Autodesk Inventor part; units mm, degrees
ref_plane "YZ Plane" through (0, 0, 0) normal (1, 0, 0) x (0, 1, 0)
ref_plane "XZ Plane" through (0, 0, 0) normal (0, 1, 0) x (-1, 0, 0)
ref_plane "XY Plane" through (0, 0, 0) normal (0, 0, 1) x (1, 0, 0)
sketch "Sketch1" plane through (0, 0, 0) normal (0, 1, 0) x (-1, 0, 0)
  line L0 (100, 100.3504) -> (-94, 100.3504)
  line L1 (94, -100) -> (94, -50)
  line L2 (94, -50) -> (100, -50)
  line L3 (100, 0) -> (94, 0)
  line L4 (-100, -50) -> (-94, -50)
  line L5 (-94, -50) -> (-94, 0)
  line L6 (-94, 0) -> (-100, 0)
  line L7 (94, 0) -> (94, 50)
  line L8 (94, 50) -> (100, 50)
  line L9 (94, 0) -> (100, 0)
  line L10 (-100, 50) -> (-94, 50)
  line L11 (-94, 50) -> (-94, 100.3504)
  line L12 (94, -100) -> (-100, -100)
  line L13 (100, -50) -> (100, 0)
  line L14 (100, 50) -> (100, 100.3504)
  line L15 (-100, 50) -> (-100, 0)
  line L16 (-100, -50) -> (-100, -100)
  point P0 (0, 0)
  dimension "d23" = 50
  dimension "d25" = 6
  dimension "d26" = 50
  dimension "d27" = 50
extrude "Extrusion2" add sketch "Sketch1" along normal blind 6
properties part number "simple wall test"
Model file for the job. Use its own axes, mm. A direction names the side the tool comes from. Coordinates: 2 decimals unless noted, no trailing zeros. Write each loop counter-clockwise with the first axis right and the second up, starting at its lowest first coordinate (ties: lowest second). Pieces come first, ordered by that corner, then holes. Notation, with made-up numbers: (0, -35.5) - (52, -35.5) arc R36 cw to (52, 0.5) - close; hole circle Ø4 at (70.5, 3). An arc over 180 degrees is marked (long way). Use a Markdown table: item, result. Add a question column.
Item 1: Drop flat-ended pins along their axis: pin 1 (3 mm diameter, centred on x = 97, y = 3.5, fed in from +Z); pin 2 (3 mm diameter, centred on y = 3.5, z = 17.5, fed in from -X); pin 3 (1.8 mm diameter, centred on x = -96.5, y = 2.5, fed in from -Z). Give the stop position or say it passes through.
Item 2: Drill centre lines: line 1 along X through (y, z) = (1.7, -84); line 2 along X through (y, z) = (2.85, 63.5). Where is each one in solid material? Low to high.
Item 3: Band-saw the part on B-B, the plane z = -68. Write the cut outline in (x, y), and give its area (3 significant figures).
Item 4: 3-axis set-ups, long thin cutter, end or side, ignore diameter. For faces 1 (the face through (-94, 3, -75)), 2 (the face through (97, 3, 0)), 3 (the face through (97, 3, 50)), 4 (the face through (-94, 3, 25)): which of +Z, -Z, +X, -X, +Y, -Y reach the whole face in a straight line?
Item 5: Band-saw the part on A-A, the plane y = 3.9. Write the cut outline in (x, z).
Item 6: Two-plate mould, pull along Z, no slides. Class faces 5 (the face through (97, 3, -50)), 6 (the face through (100, 3, -75)), 7 (the face through (2, 3, -100)): pulls with the +Z half, pulls with the -Z half, needs draft (parallel to the pull), parting line crosses it, or undercut.
A:
| question | item | result |
|---|---|---|
| 1 | pin 1 | stops at z = 50 |
| 1 | pin 2 | stops at x = -94 |
| 1 | pin 3 | stops at z = -50 |
| 2 | line 1 | x = -94 to 100 |
| 2 | line 2 | x = -100 to 94 |
| 3 | outline | (-94, 0) - (100, 0) - (100, 6) - (-94, 6) - close |
| 3 | area | 1,160 mm² |
| 4 | face 1 | -Z, -X, +Y, -Y |
| 4 | face 2 | +X, +Y, -Y |
| 4 | face 3 | +Z, +X, +Y, -Y |
| 4 | face 4 | -X, +Y, -Y |
| 5 | outline | (-100, -50) - (-94, -50) - (-94, -100) - (100, -100) - (100, -50) - (94, -50) - (94, 0) - (100, 0) - (100, 50) - (94, 50) - (94, 100.35) - (-100, 100.35) - (-100, 50) - (-94, 50) - (-94, 0) - (-100, 0) - close |
| 6 | face 5 | undercut |
| 6 | face 6 | needs draft |
| 6 | face 7 | pulls with the -Z half |
